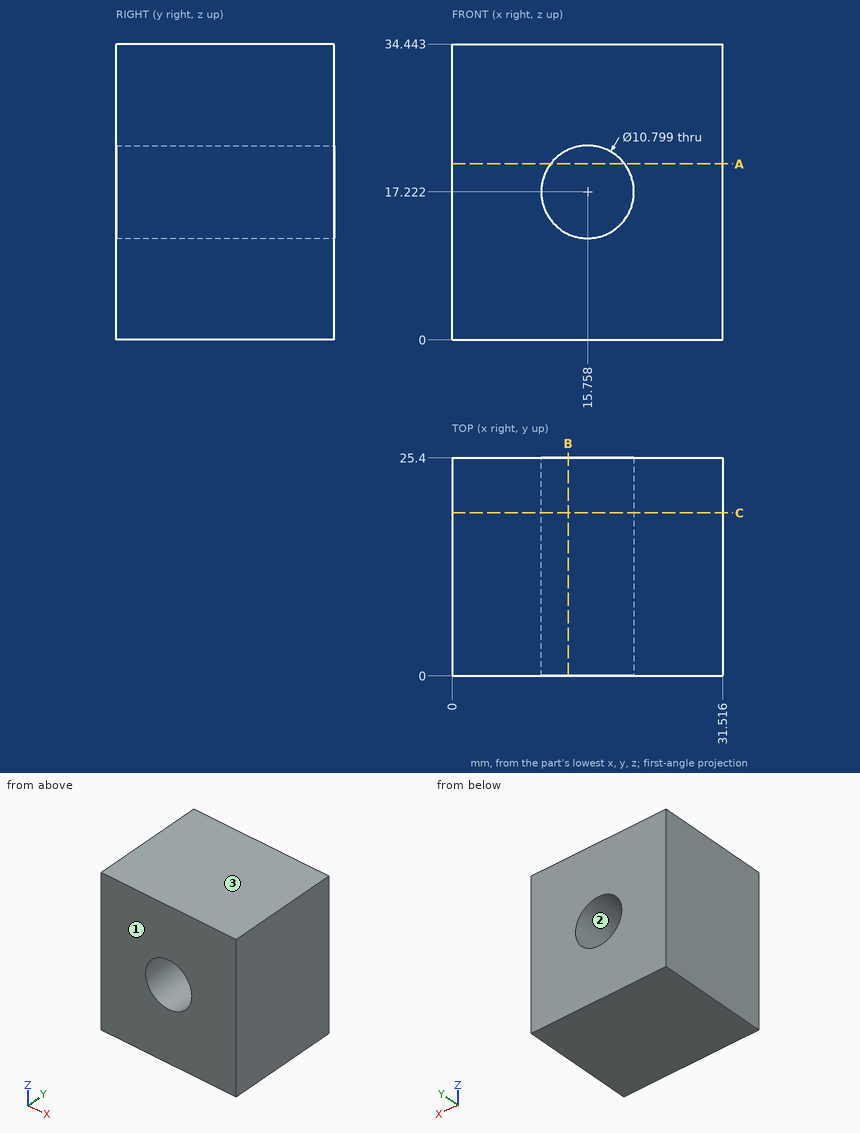
The drawing under review shows one solid part. Ordinate dimensions are in mm from its lowest x, y, z. Round coordinates to 2 decimals unless told otherwise and drop trailing zeros. Order: outer loops, then holes, each group sorted by start corner. A loop starts at its lowest first (then second) coordinate and runs counter-clockwise, first axis right, second up. Notation, with made-up numbers: (16.25, 18) -> (33.25, 18) arc R12 ccw to (33.25, 23) -> close; hole circle Ø11 at (-15.5, 45). An arc over 180 degrees is marked (long way). Return JSON: item names as keys, results as strings.
1. Take a section at C-C (y = 19). Write out the cut boundary in (x, z), then the cut area to 3 significant figures.
Answer block:
{"outline": "(0, 0) -> (31.52, 0) -> (31.52, 34.44) -> (0, 34.44) -> close; hole circle Ø10.8 at (15.76, 17.22)", "area": "994 mm²"}
2. For L1, parallel to X at y = 6.75, z = 20 (1 decimal); L2, parallel to Z at x = 11, y = 13.75 (1 decimal); L3, parallel to X at y = 5.5, z = 16, list the stretches that pass through material, from the lowest coordinate up. Write a range as [from, to].
Answer block:
{"L1": "x = [0, 11.1], [20.4, 31.5]", "L2": "z = [0, 14.7], [19.8, 34.4]", "L3": "x = [0, 10.5], [21.02, 31.52]"}
3. Take a section at A-A (z = 20.5). Write out the cut boundary in (x, y).
Answer block:
{"outline": "(0, 0) -> (11.47, 0) -> (11.47, 25.4) -> (0, 25.4) -> close; (20.05, 0) -> (31.52, 0) -> (31.52, 25.4) -> (20.05, 25.4) -> close"}
4. Insertion check: P1, Ø5, axis at y = 5.5, z = 9, coming from the -X side; P2, Ø9.5, axis at x = 15.76, z = 17.22, coming from the +Y side. Each pin has a flat end and moves straight along its axis. Give the tip position at first contact, or say it passes through.
Answer block:
{"P1": "stops at x = 0", "P2": "passes through"}
5. Take a section at B-B (x = 13.5). Write out the cut boundary in (y, z), then the cut area to 3 significant figures.
Answer block:
{"outline": "(0, 0) -> (25.4, 0) -> (25.4, 12.32) -> (0, 12.32) -> close; (0, 22.13) -> (25.4, 22.13) -> (25.4, 34.44) -> (0, 34.44) -> close", "area": "626 mm²"}
6. The part is to be moulded in two halves that separate along Z. For the marked faces 1, 2 and 3, say which applies: +Z half, -Z half, draft (parallel to the pull), parting line (faces both ways), or undercut.
Answer block:
{"face 1": "draft", "face 2": "undercut", "face 3": "+Z half"}
